from build123d import *

# Parameters (mm, degrees)
F0_W     = 33
F0_H     = 25
F1_DEPTH = 25
F2_R     = 3.5
F3_DEPTH = 25.001
F4_R     = 3.75
F5_DEPTH = 33.001


with BuildPart() as f1:
    # F0 (on Front) → F1 (new body)
    with BuildSketch(Plane.XZ):
        with Locations((16.5, 12.5)):
            Rectangle(F0_W, F0_H)
    extrude(amount=F1_DEPTH)

    # F2 (on Top) → F3 (cut, through all)
    with BuildSketch(Plane.XY):
        with Locations((16.5, -16.25)):
            Circle(F2_R)
    extrude(amount=F3_DEPTH, mode=Mode.SUBTRACT)

    # F4 (on Right) → F5 (cut, through all)
    with BuildSketch(Plane.YZ):
        with Locations((-8.5, 12.5)):
            Circle(F4_R)
    extrude(amount=F5_DEPTH, mode=Mode.SUBTRACT)


solid = f1.part
Design review of the part built by this model. Coordinates are the model's own, in mm. Give positions to 0.01 mm unless a question says otherwise; leave off trailing zeros. Write each loop counter-clockwise with the first axis right and the second up, starting at its lowest first coordinate (ties: lowest second). Pieces come first, ordered by that corner, then holes. Notation, with made-up numbers: M 15,-3.75 L 45,-3.75 A17 cw 45,7.25 Z; hole C 15,-29.5 d8. An arc over 180 degrees is marked long. Return JSON: item names as keys, results as strings. Group by question number.
Item 1: The part is to be moulded in two halves that separate along Z. For faces 1 (the cylindrical face through (16.269, -11.264, 15.034)), 2 (the flat face through (16, -12, 25)), 3 (the flat face through (16, -12, 0)), 4 (the flat face through (16, 0, 13)), say which applies: pulls with the +Z half, pulls with the -Z half, needs draft (parallel to the pull), parting line crosses it, or undercut.
Item 2: Wall thickness on line 1 along X through (y, z) = (-16.25, 5.25); line 2 along Y through (x, z) = (19.5, 11); line 3 along Y through (x, z) = (16.5, 9.5): over which ranges is each line inside the solid? List them lowest first.
Item 3: Take a section at A-A (z = 14.75). Give the boundary of the cut face in (x, y).
Item 4: Take a section at D-D (z = 21). Give the boundary of the cut face in (x, y), plus the area to 3 significant figures.
Item 5: Clearance check with a flat-ended pin moving along its axis: pin 1 Ø3 at (x, y) = (17, -17) entering from -Z. State where the tip first meets the part, or that it passes through.
Item 6: Take a section at C-C (y = -16.25). Give the boundary of the cut face in (x, z), plus the area to 3 significant figures.
Item 7: Take a section at B-B (x = 16.5). Give the boundary of the cut face in (y, z), plus the area to 3 significant figures.
Return value:
{
 "1": {"face 1": "undercut", "face 2": "pulls with the +Z half", "face 3": "pulls with the -Z half", "face 4": "needs draft"},
 "2": {"line 1": "x = 0 to 13, 20 to 33", "line 2": "y = -25 to -18.05, -14.45 to -11.94, -5.06 to 0", "line 3": "y = -25 to -19.75, -12.75 to -10.75, -6.25 to 0"},
 "3": {"outline": "M 0,-25 L 33,-25 L 33,-11.5 L 0,-11.5 Z; M 0,-5.5 L 33,-5.5 L 33,0 L 0,0 Z; hole C 16.5,-16.25 d7"},
 "4": {"outline": "M 0,-25 L 33,-25 L 33,0 L 0,0 Z; hole C 16.5,-16.25 d7", "area": "787 mm2"},
 "5": {"pin 1": "passes through"},
 "6": {"outline": "M 0,0 L 13,0 L 13,25 L 0,25 Z; M 20,0 L 33,0 L 33,25 L 20,25 Z", "area": "650 mm2"},
 "7": {"outline": "M -25,0 L -19.75,0 L -19.75,25 L -25,25 Z; M -12.75,0 L 0,0 L 0,25 L -12.75,25 Z; hole C -8.5,12.5 d7.5", "area": "406 mm2"}
}
